Check sheet for the modelled part. Datum: model origin and axes. Units: mm. A direction names the side the tool comes from. Give positions to 0.01 mm unless a question says otherwise; leave off trailing zeros.
```python
from build123d import *

# Parameters (mm, degrees)
F0_R      = 25
F1_DEPTH  = 25
F5_R      = 25
F6_DEPTH  = 5
F8_DEPTH  = 4
F9_R      = 3
F10_DEPTH = 25


with BuildPart() as f1:
    # F0 (on Top) → F1 (new body)
    with BuildSketch(Plane.XY):
        Circle(F0_R)
    extrude(amount=F1_DEPTH)

    # F3 (on face) → F4 section 0
    with BuildSketch(Plane.XY.offset(25)):
        Polygon((-3.4807621135, 12.9903810568), (-7.5, 12.9903810568), (-9.5096189432, 9.5096189432), (-12.9903810568, 7.5), (-12.9903810568, 3.4807621135), (-15, 0), (-12.9903810568, -3.4807621135), (-12.9903810568, -7.5), (-9.5096189432, -9.5096189432), (-7.5, -12.9903810568), (-3.4807621135, -12.9903810568), (0, -15), (3.4807621135, -12.9903810568), (7.5, -12.9903810568), (9.5096189432, -9.5096189432), (12.9903810568, -7.5), (12.9903810568, -3.4807621135), (15, 0), (12.9903810568, 3.4807621135), (12.9903810568, 7.5), (9.5096189432, 9.5096189432), (7.5, 12.9903810568), (3.4807621135, 12.9903810568), (0, 15), align=None)
    # F2 (on face) → F4 section 1
    with BuildSketch(Plane(origin=(0, 0, 0), x_dir=(1, 0, 0), z_dir=(0, 0, -1))):
        Polygon((-4.9102076485, 20), (-11.5470053838, 20), (-14.414081985, 15.0340776575), (-19.4962760907, 12.3785520935), (-19.7756118999, 5.7476354385), (-23.0940107676, 0), (-20.2269341664, -4.9659223425), (-20.4682786203, -10.694994327), (-14.8654042514, -14.2523645615), (-11.5470053838, -20), (-5.8128521814, -20), (-0.9720025297, -23.0735464204), (4.9102076485, -20), (11.5470053838, -20), (14.414081985, -15.0340776575), (19.4962760907, -12.3785520935), (19.7756118999, -5.7476354385), (23.0940107676, 0), (20.2269341664, 4.9659223425), (20.4682786203, 10.694994327), (14.8654042514, 14.2523645615), (11.5470053838, 20), (5.8128521814, 20), (0.9720025297, 23.0735464204), align=None)
    loft(mode=Mode.SUBTRACT)

    # F5 (on face) → F6 (join)
    with BuildSketch(Plane.XY.offset(25)):
        Circle(F5_R)
    extrude(amount=F6_DEPTH)

    # F7 (on face) → F8 (cut)
    with BuildSketch(Plane(origin=(0, 0, 25), x_dir=(1, 0, 0), z_dir=(0, 0, -1))):
        Polygon((2.8867513459, 5), (-2.8867513459, 5), (-5.7735026919, 0), (-2.8867513459, -5), (2.8867513459, -5), (5.7735026919, 0), align=None)
    extrude(amount=-F8_DEPTH, mode=Mode.SUBTRACT)

    # F9 (on face) → F10 (cut)
    with BuildSketch(Plane.XY.offset(30)):
        Circle(F9_R)
    extrude(amount=-F10_DEPTH, mode=Mode.SUBTRACT)


solid = f1.part
```
Q1. Material ranges on line 1 (Y direction, x = 0, z = 29.3); line 2 (Z direction, x = 11, y = 1.5); line 3 (Y direction, x = 5, z = 6), recorded low to high.
Q2. Tool access check on faces 4 (the flat face through (0, -5, 27)), 5 (the cylindrical face through (-3, 0.1, 29.5)). Record the directions out of +Z, -Z, +X, -X, +Y, -Y that give a thin tool (end or side, any length) a straight path to the whole face; none if there is none.
Q3. Go/stop test with flat-tipped pins: P1, Ø9.5, axis at x = 0, y = 0, coming from the +Z side; P2, Ø10, axis at x = 17.5, z = 14.5, coming from the -Y side; P3, Ø2, axis at x = 1.5, z = 26, coming from the +Y side (3 decimals); P4, Ø1.5, axis at x = 0.5, z = 18, coming from the -Y side. Record where each tip stops, or that it passes through.
Q4. Draft check along Y on faces 1 (the cylindrical face through (23.846, 7.509, 14.79)), 2 (the flat face through (0, -5, 30)), 3 (the flat face through (0, 5, 27)). Enter one of: pulls with the +Y half, pulls with the -Y half, needs draft (parallel to the pull), parting line crosses it, or undercut.
Filled in:
1. line 1: y = -25 to -3, 3 to 25
1. line 2: z = 25 to 30
1. line 3: y = -24.49 to -18.48, 18.32 to 24.49
2. face 4: -Z
2. face 5: +Z, -Z
3. P1: stops at z = 30
3. P2: stops at y = -21.65
3. P3: stops at y = 24.995
3. P4: stops at y = -25
4. face 1: parting line crosses it
4. face 2: needs draft
4. face 3: undercut
